Autodesk Inventor part; units mm, degrees
ref_plane "YZ Plane" through (0, 0, 0) normal (1, 0, 0) x (0, 1, 0)
ref_plane "XZ Plane" through (0, 0, 0) normal (0, 1, 0) x (-1, 0, 0)
ref_plane "XY Plane" through (0, 0, 0) normal (0, 0, 1) x (1, 0, 0)
sketch "Sketch1" plane through (0, 0, 0) normal (0, 0, 1) x (1, 0, 0)
  circle A0 centre (0, 0) radius 15
  circle A1 centre (0, 0) radius 20
  circle A2 centre (0, 0) radius 32.5
  circle A3 centre (0, 0) radius 50
  dimension "d0" = 30
  dimension "d1" = 40
  dimension "d2" = 65
  dimension "d3" = 100
extrude "Extrusion1" add sketch "Sketch1" along normal blind 10 contours A2 | A3
extrude "Extrusion2" add sketch "Sketch1" along normal blind 20 contours A1
extrude "Extrusion3" add sketch "Sketch1" along normal blind 15 contours A2
fillet "Fillet1" radius 5 1 edges at (-20, 0, 15)
extrude "Extrusion4" cut sketch "Sketch1" along normal blind 2 contours A1 | A2
sketch "Sketch3" plane through (0, 0, 10) normal (0, 0, 1) x (1, 0, 0)
  point P0 (41, 0)
  point P1 (0, 41)
  point P2 (-28.9914, 28.9914)
  point P3 (-41, 0)
  point P4 (-28.9914, -28.9914)
  point P5 (0, -41)
  point P6 (28.9914, -28.9914)
  point P7 (28.9914, 28.9914)
hole "Hole2" at (41, 0, 10) at (0, 41, 10) at (-28.9914, 28.9914, 10) at (-41, 0, 10) at (-28.9914, -28.9914, 10) at (0, -41, 10) at (28.9914, -28.9914, 10) at (28.9914, 28.9914, 10) direction (0, 0, -1) diameter 9 end through all
Design review of the part built by this model. Coordinates are the model's own, in mm. A direction names the side the tool comes from. Round coordinates to 2 decimals unless told otherwise and drop trailing zeros. Write each loop counter-clockwise with the first axis right and the second up, starting at its lowest first coordinate (ties: lowest second). Pieces come first, ordered by that corner, then holes. Notation, with made-up numbers: (59.5, 45.5) - (64.5, 45.5) arc R19 cw to (64.5, 67.5) - close; hole circle Ø6 at (47.25, 18.5). An arc over 180 degrees is marked (long way). Return JSON: item names as keys, results as strings. Group by question number.
Item 1: Machinability: for faces 4 (the face through (31, -9.76, 0.99)), 5 (the face through (31.73, 32.56, 4.93)), 6 (the face through (17, -19, 15)), which of the approach directions +Z, -Z, +X, -X, +Y, -Y give a long, thin tool a straight path to every point of the face, cutting with its end or side? Answer none if there is none.
Item 2: We need section D-D on z = 13.25. Write out the cut boundary in (x, y).
Item 3: We need section C-C on x = -42.5. Write out the cut boundary in (y, z).
Item 4: For probe 1 along Y at (x, z) = (0, 7.5); probe 2 along X at (y, z) = (-26, 3.25); probe 3 along Y at (x, z) = (-27, 5), list the stretches that pass through material, from the lowest coordinate up. Write a range as [from, to].
Item 5: The part is to be moulded in two halves that separate along Y. For faces 1 (the face through (-33.453, -28.406, 4.93)), 2 (the face through (-1, -33, 0)), 3 (the face through (31, -9.76, 12.46)), say which applies: pulls with the +Y half, pulls with the -Y half, needs draft (parallel to the pull), parting line crosses it, or undercut.
Item 6: Insertion check: P1, Ø12, axis at y = -5, z = 10.5, coming from the +X side; P2, Ø1.5, axis at y = 14, z = 4, coming from the +X side; P3, Ø4, axis at x = 1.5, y = 16.5, coming from the -Z side; P4, Ø1, axis at x = 26, y = -23.5, coming from the +Z side. Each pin has a flat end and moves straight along its axis. Give the tip position at first contact, or say it passes through.
Item 7: We need section A-A on y = 0. Give the number of separate pieces and of enclosed holes in the cut face, and give its area (3 significant figures).
Model answer:
{
 "1": {"face 4": "-Z", "face 5": "+Z, -Z", "face 6": "+Z"},
 "2": {"outline": "circle Ø65 at (0, 0); hole circle Ø30 at (0, 0)"},
 "3": {"outline": "(-26.34, 0) - (-4.24, 0) - (-4.24, 10) - (-26.34, 10) - close; (4.24, 0) - (26.34, 0) - (26.34, 10) - (4.24, 10) - close"},
 "4": {"probe 1": "y = [-50, -45.5], [-36.5, -15], [15, 36.5], [45.5, 50]", "probe 2": "x = [-42.71, -32.35], [-25.63, 25.63], [32.35, 42.71]", "probe 3": "y = [-42.08, -33.03], [-24.96, 24.96], [33.03, 42.08]"},
 "5": {"face 1": "undercut", "face 2": "needs draft", "face 3": "parting line crosses it"},
 "6": {"P1": "stops at x = 50", "P2": "stops at x = 48.21", "P3": "stops at z = 2", "P4": "stops at z = 10"},
 "7": {"separate pieces": "4", "enclosed holes": "0", "area": "686 mm²"}
}
